Design review of the part built by this model. Coordinates are the model's own, in mm. A direction names the side the tool comes from. Round coordinates to 2 decimals unless told otherwise and drop trailing zeros. Order: outer loops, then holes, each group sorted by start corner. A loop starts at its lowest first (then second) coordinate and runs counter-clockwise, first axis right, second up. Notation, with made-up numbers: M 76.5,-30 L 103.5,-30 A28 ccw 103.5,4 Z; hole C 35.5,74 d4. An arc over 180 degrees is marked long. Write each question's results on one line, items separated by ' | '. Start each with the question number.
Item 1: Machinability: for faces 4 (the flat face through (4, 5, -1)), 5 (the cylindrical face through (5.29, -2.49, -0.04)), 6 (the flat face through (5, 2, 2)), 7 (the cylindrical face through (6.64, -2.49, -2.1)), which of the approach directions +Z, -Z, +X, -X, +Y, -Y give a long, thin tool a straight path to every point of the face, cutting with its end or side? Answer none if there is none.
Item 2: Take a section at A-A, the plane y = 4.75. Write out the cut boundary in (x, z), plus the area to 3 significant figures.
Item 3: Take a section at D-D, the plane z = 0.25. Write out the cut boundary in (x, y), plus the area to 3 significant figures.
Item 4: The part is to be moulded in two halves that separate along X. For faces 1 (the flat face through (5.2, -1.502, -1.3)), 2 (the cylindrical face through (2.36, 1.46, -5.2)), 3 (the cylindrical face through (3.68, 1.43, -3.66)), say which applies: +X half, -X half, draft (parallel to the pull), parting line (faces both ways), or undercut.
Item 5: Clearance check with flat-ended pins moving along their axes: pin 1 (2 mm diameter, centred on x = 7, z = -3.5, fed in from +Y); pin 2 (1.4 mm diameter, centred on x = 4.5, z = -0.45, fed in from +Y); pin 3 (2.5 mm diameter, centred on x = 3.5, y = 5, fed in from -Z); pin 4 (1.1 mm diameter, centred on x = 4.5, z = -4, fed in from +Y). State where each tip first meets the part, or that it passes through.
Item 6: Wall thickness on line 1 (Z direction, x = 4.5, y = 1.5); line 2 (Y direction, x = 4.3, z = -2); line 3 (Z direction, x = 4.5, y = -2.1): over which ranges is each line inside the solid? List them lowest first. Write a range as [from, to].
Item 7: Take a section at C-C, the plane z = -2.5. Write out the cut boundary in (x, y).
```python
from build123d import *

# Parameters (mm, degrees)
BOSS_EXTRUDE1_DEPTH       = 6
SKETCH3_W                 = 7.6
SKETCH3_H                 = 16
CUT_EXTRUDE2_DEPTH        = 11.990294347
CUT_EXTRUDE3_DEPTH        = 11.990294347
FILLET2_R                 = 3
FILLET3_R                 = 0.5
F_2_56_TAPPED_HOLE1_D     = 1.778
F_2_56_TAPPED_HOLE1_DEPTH = 3
F_2_56_TAPPED_HOLE1_TIP   = 0.53416509
SKETCH13_R                = 0.5
CUT_EXTRUDE10_DEPTH       = 10


# Some blends are built 0.0001 mm under size
with BuildPart() as part:
    # Sketch1 → Boss-Extrude1 (new body)
    with BuildSketch(Plane(origin=(7.5, 0, 0), x_dir=(0, 0, -1), z_dir=(1, 0, 0))):
        with BuildLine():
            Line((-2, 0.497577099), (-2, 5.397577099))
            ThreePointArc((-2, 5.397577099), (-1.5, 5.897577099), (-1, 5.397577099))
            Line((-1, 5.397577099), (-1, 0.497577099))
            Line((-1, 0.497577099), (6.1, 0.497577099))
            Line((6.1, 0.497577099), (6.1, 6.897577099))
            Line((6.1, 6.897577099), (-2.9, 6.897577099))
            Line((-2.9, 6.897577099), (-2.9, -3.502422901))
            Line((-2.9, -3.502422901), (3, -3.502422901))
            Line((3, -3.502422901), (3, -1.502422901))
            Line((3, -1.502422901), (-2, -1.502422901))
            Line((-2, -1.502422901), (-2, 0.497577099))
        make_face()
    extrude(amount=-BOSS_EXTRUDE1_DEPTH)

    # Sketch3 → Cut-Extrude2 (cut, through all)
    with BuildSketch(Plane.ZY.offset(-1.5)):
        with Locations((6.8, 14.497577099)):
            Rectangle(SKETCH3_W, SKETCH3_H)
        with Locations((-3.7, 14.497577099)):
            Rectangle(SKETCH3_W, SKETCH3_H)
    extrude(amount=-CUT_EXTRUDE2_DEPTH, mode=Mode.SUBTRACT)

    # Sketch4 → Cut-Extrude3 (cut, through all)
    with BuildSketch(Plane.ZY.offset(-1.5)):
        Polygon((-1.707106781, 2.397577099), (-1, 2.397577099), (-1, 3.20468388), (-1, 6.497577099), (-7.5, 6.497577099), (-7.5, 2.397577099), align=None)
    extrude(amount=-CUT_EXTRUDE3_DEPTH, mode=Mode.SUBTRACT)

    # Fillet2
    fillet2_edges = [part.edges().sort_by_distance(p)[0] for p in [
        (7.5, 1.447577099, -6.1),
        (1.5, 1.447577099, -6.1),
        (7.5, -2.502422901, -3),
        (1.5, -2.502422901, -3),
    ]]
    fillet(fillet2_edges, radius=FILLET2_R - 0.0001)  # a hair under: the kernel refuses the full size

    # Fillet3
    # the kernel refuses this fillet: 0.5 mm, written as the material it adds along each edge
    with BuildSketch(Plane(origin=(1.5, 6.497577099, 0.1), x_dir=(0, 1.0, -1.570583940679385e-12), z_dir=(1, 0, 0))) as fillet3_piece_1:
        with BuildLine():
            CenterArc((0.5, -0.489897949), FILLET3_R, 101.536959033, 78.463040967)
            Line((0, -0.489897949), (-0.01, -0.489897949))
            Line((-0.01, -0.489897949), (-0.01, 0))
            Line((-0.01, 0), (0, 0.01))
            ThreePointArc((0, 0.01), (0.2, 0.01), (0.398, 0.009797959))
            Line((0.398, 0.009797959), (0.4, 0))
        make_face()
    extrude(amount=6)
    with BuildSketch(Plane(origin=(7.5, -1.502422901, 2), x_dir=(0, 0, -1), z_dir=(-1, 0, 0))) as fillet3_piece_2:
        with BuildLine():
            CenterArc((FILLET3_R, -FILLET3_R), FILLET3_R, 90, 90)
            Line((0, -FILLET3_R), (-FILLET3_R * 0.02, -FILLET3_R))
            Line((-FILLET3_R * 0.02, -FILLET3_R), (-FILLET3_R * 0.02, FILLET3_R * 0.02))
            Line((-FILLET3_R * 0.02, FILLET3_R * 0.02), (FILLET3_R, FILLET3_R * 0.02))
            Line((FILLET3_R, FILLET3_R * 0.02), (FILLET3_R, 0))
        make_face()
    extrude(amount=6)

    # #2-56 Tapped Hole1
    with Locations(Plane(origin=(0, 2.397577099, 0), x_dir=(1, 0, 0), z_dir=(0, 1, 0))):
        with Locations((4.5, 4)):
            Hole(F_2_56_TAPPED_HOLE1_D / 2, depth=F_2_56_TAPPED_HOLE1_DEPTH)
            with Locations((0, 0, -(F_2_56_TAPPED_HOLE1_DEPTH + F_2_56_TAPPED_HOLE1_TIP / 2))):  # 118° drill point
                Cone(0, F_2_56_TAPPED_HOLE1_D / 2, F_2_56_TAPPED_HOLE1_TIP, mode=Mode.SUBTRACT)

    # Sketch12 → #2-56 Tapped Hole2 (revolve, cut)
    with BuildSketch(Plane(origin=(4.5, -1.502422901, -0.45), x_dir=(0, 0, 1), z_dir=(1, 0, 0))):
        Polygon((0, 0), (0, 5.87416509), (0.889, 5.34), (0.889, 0), align=None)
    revolve(axis=Axis((4.5, 4.847577099, -0.45), (0, -1, 0)), mode=Mode.SUBTRACT)

    # Sketch13 → Cut-Extrude10 (cut)
    with BuildSketch(Plane.ZY.offset(-1.5)):
        with Locations((-1.282842712, 2.680419811)):
            Circle(SKETCH13_R)
    extrude(amount=-CUT_EXTRUDE10_DEPTH, mode=Mode.SUBTRACT)


solid = part.part
```
Results list:
1) face 4: -Z, +X, -X, +Y | face 5: -Y | face 6: +X, -X | face 7: -Z, +X, -Y
2) outline: M 1.5,-1 L 7.5,-1 L 7.5,1 L 1.5,1 Z; M 1.5,2 L 7.5,2 L 7.5,2.9 L 1.5,2.9 Z | area: 17.4 mm²
3) outline: M 1.5,-3.5 L 3.95,-3.5 L 3.95,-1.5 L 1.5,-1.5 Z; M 1.5,0.5 L 7.5,0.5 L 7.5,6.9 L 1.5,6.9 Z; M 5.05,-3.5 L 7.5,-3.5 L 7.5,-1.5 L 5.05,-1.5 Z | area: 48.2 mm²
4) face 1: draft | face 2: -X half | face 3: undercut
5) pin 1: y = 2.4 | pin 2: y = 6.9 | pin 3: z = -1 | pin 4: through
6) line 1: [-6.1, -4.89], [-3.11, 1], [2, 2.9] | line 2: [-3.5, -1.5], [0.5, 2.4] | line 3: [-3, -1.34], [0.44, 2.9]
7) outline: M 1.5,0.5 L 7.5,0.5 L 7.5,2.4 L 1.5,2.4 Z; M 2.84,-3.5 L 6.16,-3.5 L 6.16,-1.5 L 2.84,-1.5 Z
